```python
from build123d import *

# Parameters (mm, degrees)
BASE_FLANGE1_DEPTH        = 130
UNFOLD1_DEPTH             = 130
UNFOLD1_2_DEPTH           = 130
SKETCH6_W                 = 0.3
SKETCH6_H                 = 8
CUT_EXTRUDE1_DEPTH        = 235.985371885
LPATTERN1_COUNT           = 3
LPATTERN1_PITCH           = 11
LPATTERN2_COUNT           = 3
LPATTERN2_PITCH           = 100
LPATTERN2_COPY_1_SKETCH_W = 0.3
LPATTERN2_COPY_1_SKETCH_H = 8
LPATTERN2_COPY_1_DEPTH    = 235.985371885
LPATTERN2_COPY_2_SKETCH_W = 0.3
LPATTERN2_COPY_2_SKETCH_H = 8
LPATTERN2_COPY_2_DEPTH    = 235.985371885
LPATTERN2_COPY_3_SKETCH_W = 0.3
LPATTERN2_COPY_3_SKETCH_H = 8
LPATTERN2_COPY_3_DEPTH    = 235.985371885
LPATTERN2_COPY_4_SKETCH_W = 0.3
LPATTERN2_COPY_4_SKETCH_H = 8
LPATTERN2_COPY_4_DEPTH    = 235.985371885
FOLD1_DEPTH               = 130
FOLD1_2_DEPTH             = 130
FOLD1_START               = 30
FOLD1_3_DEPTH             = 70
FOLD1_START_2             = 8
FOLD1_4_DEPTH             = 3
FOLD1_START_3             = 19
FOLD1_5_DEPTH             = 3
FOLD1_START_4             = 108
FOLD1_6_DEPTH             = 3
FOLD1_START_5             = 119
FOLD1_7_DEPTH             = 3


# Read off the part's stored shape, not the designer's step: Unfold1, Fold1
# Sheet-metal steps are written as plain solids
with BuildPart() as part:
    # Sketch1 → Base-Flange1 (new body)
    with BuildSketch(Plane(origin=(0, 0, 0), x_dir=(1, 0, 0), z_dir=(0, 1, 0))):
        with BuildLine():
            ThreePointArc((195.5, 0), (194.920264754, 15.044613261), (193.184497308, 30))
            Line((193.184497308, 30), (193.431536307, 30.038363171))
            ThreePointArc((193.431536307, 30.038363171), (195.169523405, 15.063851897), (195.75, 0))
            Line((195.75, 0), (195.5, 0))
        make_face()
    extrude(amount=BASE_FLANGE1_DEPTH)

    # Unfold1 outline → Unfold1 (cut)
    with BuildSketch(Plane(origin=(0, 0, 0), x_dir=(1, 0, 0), z_dir=(0, 1, 0))):
        with BuildLine():
            Line((195.5, 0), (195.5, 9.890020227))
            ThreePointArc((195.5, 9.890020227), (194.726536236, 19.990962601), (193.431536307, 30.038363171))
            Line((193.431536307, 30.038363171), (193.184497308, 30))
            ThreePointArc((193.184497308, 30), (194.920264754, 15.044613261), (195.5, 0))
        make_face()
    extrude(amount=UNFOLD1_DEPTH, mode=Mode.SUBTRACT)

    # Unfold1 2 outline → Unfold1 2 (add)
    with BuildSketch(Plane(origin=(0, 0, 0), x_dir=(1, 0, 0), z_dir=(0, 1, 0))):
        with BuildLine():
            Line((195.75, 0), (195.75, 30.138261696))
            Line((195.75, 30.138261696), (195.5, 30.138261696))
            Line((195.5, 30.138261696), (195.5, 9.890020227))
            ThreePointArc((195.5, 9.890020227), (195.687490019, 4.946589737), (195.75, 0))
        make_face()
    extrude(amount=UNFOLD1_2_DEPTH)

    # Sketch6 → Cut-Extrude1 (cut, symmetric)
    with BuildSketch(Plane(origin=(195.75, 0, -195.75), x_dir=(0, 0, 1), z_dir=(-1, 0, 0))):
        with Locations((175.6, 126)):
            Rectangle(SKETCH6_W, SKETCH6_H)
    cut_extrude1 = extrude(amount=CUT_EXTRUDE1_DEPTH, both=True, mode=Mode.SUBTRACT)

    # LPattern1: Cut-Extrude1 ×3
    with Locations(*[(0, -i * LPATTERN1_PITCH, 0) for i in range(1, LPATTERN1_COUNT)]):
        add(cut_extrude1, mode=Mode.SUBTRACT)

    # LPattern2: Cut-Extrude1 ×3
    with Locations(*[(0, -i * LPATTERN2_PITCH, 0) for i in range(1, LPATTERN2_COUNT)]):
        add(cut_extrude1, mode=Mode.SUBTRACT)

    # LPattern2 copy 1 sketch → LPattern2 copy 1 (cut, symmetric)
    with BuildSketch(Plane(origin=(195.75, -111, -195.75), x_dir=(0, 0, 1), z_dir=(-1, 0, 0))):
        with Locations((175.6, 126)):
            Rectangle(LPATTERN2_COPY_1_SKETCH_W, LPATTERN2_COPY_1_SKETCH_H)
    extrude(amount=LPATTERN2_COPY_1_DEPTH, both=True, mode=Mode.SUBTRACT)

    # LPattern2 copy 2 sketch → LPattern2 copy 2 (cut, symmetric)
    with BuildSketch(Plane(origin=(195.75, -211, -195.75), x_dir=(0, 0, 1), z_dir=(-1, 0, 0))):
        with Locations((175.6, 126)):
            Rectangle(LPATTERN2_COPY_2_SKETCH_W, LPATTERN2_COPY_2_SKETCH_H)
    extrude(amount=LPATTERN2_COPY_2_DEPTH, both=True, mode=Mode.SUBTRACT)

    # LPattern2 copy 3 sketch → LPattern2 copy 3 (cut, symmetric)
    with BuildSketch(Plane(origin=(195.75, -122, -195.75), x_dir=(0, 0, 1), z_dir=(-1, 0, 0))):
        with Locations((175.6, 126)):
            Rectangle(LPATTERN2_COPY_3_SKETCH_W, LPATTERN2_COPY_3_SKETCH_H)
    extrude(amount=LPATTERN2_COPY_3_DEPTH, both=True, mode=Mode.SUBTRACT)

    # LPattern2 copy 4 sketch → LPattern2 copy 4 (cut, symmetric)
    with BuildSketch(Plane(origin=(195.75, -222, -195.75), x_dir=(0, 0, 1), z_dir=(-1, 0, 0))):
        with Locations((175.6, 126)):
            Rectangle(LPATTERN2_COPY_4_SKETCH_W, LPATTERN2_COPY_4_SKETCH_H)
    extrude(amount=LPATTERN2_COPY_4_DEPTH, both=True, mode=Mode.SUBTRACT)

    # Fold1 outline → Fold1 (cut)
    with BuildSketch(Plane(origin=(0, 0, 0), x_dir=(1, 0, 0), z_dir=(0, 1, 0))):
        with BuildLine():
            ThreePointArc((195.5, 9.890020227), (195.687490019, 4.946589737), (195.75, 0))
            Line((195.75, 0), (195.75, 30.138261696))
            Line((195.75, 30.138261696), (195.5, 30.138261696))
            Line((195.5, 30.138261696), (195.5, 9.890020227))
        make_face()
    extrude(amount=FOLD1_DEPTH, mode=Mode.SUBTRACT)

    # Fold1 2 outline → Fold1 2 (add)
    with BuildSketch(Plane(origin=(0, 0, 0), x_dir=(1, 0, 0), z_dir=(0, 1, 0))):
        with BuildLine():
            Line((194.448352042, 20.2506392), (194.697007224, 20.276535158))
            ThreePointArc((194.697007224, 20.276535158), (194.12564204, 25.165404877), (193.431536307, 30.038363171))
            Line((193.431536307, 30.038363171), (193.184497308, 30))
            ThreePointArc((193.184497308, 30), (193.877716571, 25.133265152), (194.448352042, 20.2506392))
        make_face()
        with BuildLine():
            ThreePointArc((195.5, 9.890020227), (195.179122281, 14.938966685), (194.727873277, 19.977934553))
            Line((194.727873277, 19.977934553), (194.479178675, 19.952419949))
            ThreePointArc((194.479178675, 19.952419949), (195.244627879, 9.989258456), (195.5, 0))
            Line((195.5, 0), (195.5, 9.890020227))
        make_face()
    extrude(amount=FOLD1_2_DEPTH)

    # Fold1 3 outline → Fold1 3 (add)
    with BuildSketch(Plane(origin=(0, 0, 0), x_dir=(1, 0, 0), z_dir=(0, 1, 0)).offset(FOLD1_START)):
        with BuildLine():
            ThreePointArc((194.727873277, 19.977934553), (194.712497491, 20.127240772), (194.697007224, 20.276535158))
            Line((194.697007224, 20.276535158), (194.448352042, 20.2506392))
            ThreePointArc((194.448352042, 20.2506392), (194.463822525, 20.101535484), (194.479178675, 19.952419949))
            Line((194.479178675, 19.952419949), (194.727873277, 19.977934553))
        make_face()
    extrude(amount=FOLD1_3_DEPTH)

    # Fold1 4 outline → Fold1 4 (add)
    with BuildSketch(Plane(origin=(0, 0, 0), x_dir=(1, 0, 0), z_dir=(0, 1, 0)).offset(FOLD1_START_2)):
        with BuildLine():
            ThreePointArc((194.727873277, 19.977934553), (194.712497491, 20.127240772), (194.697007224, 20.276535158))
            Line((194.697007224, 20.276535158), (194.448352042, 20.2506392))
            ThreePointArc((194.448352042, 20.2506392), (194.463822525, 20.101535484), (194.479178675, 19.952419949))
            Line((194.479178675, 19.952419949), (194.727873277, 19.977934553))
        make_face()
    extrude(amount=FOLD1_4_DEPTH)

    # Fold1 5 outline → Fold1 5 (add)
    with BuildSketch(Plane(origin=(0, 0, 0), x_dir=(1, 0, 0), z_dir=(0, 1, 0)).offset(FOLD1_START_3)):
        with BuildLine():
            ThreePointArc((194.727873277, 19.977934553), (194.712497491, 20.127240772), (194.697007224, 20.276535158))
            Line((194.697007224, 20.276535158), (194.448352042, 20.2506392))
            ThreePointArc((194.448352042, 20.2506392), (194.463822525, 20.101535484), (194.479178675, 19.952419949))
            Line((194.479178675, 19.952419949), (194.727873277, 19.977934553))
        make_face()
    extrude(amount=FOLD1_5_DEPTH)

    # Fold1 6 outline → Fold1 6 (add)
    with BuildSketch(Plane(origin=(0, 0, 0), x_dir=(1, 0, 0), z_dir=(0, 1, 0)).offset(FOLD1_START_4)):
        with BuildLine():
            ThreePointArc((194.727873277, 19.977934553), (194.712497491, 20.127240772), (194.697007224, 20.276535158))
            Line((194.697007224, 20.276535158), (194.448352042, 20.2506392))
            ThreePointArc((194.448352042, 20.2506392), (194.463822525, 20.101535484), (194.479178675, 19.952419949))
            Line((194.479178675, 19.952419949), (194.727873277, 19.977934553))
        make_face()
    extrude(amount=FOLD1_6_DEPTH)

    # Fold1 7 outline → Fold1 7 (add)
    with BuildSketch(Plane(origin=(0, 0, 0), x_dir=(1, 0, 0), z_dir=(0, 1, 0)).offset(FOLD1_START_5)):
        with BuildLine():
            ThreePointArc((194.727873277, 19.977934553), (194.712497491, 20.127240772), (194.697007224, 20.276535158))
            Line((194.697007224, 20.276535158), (194.448352042, 20.2506392))
            ThreePointArc((194.448352042, 20.2506392), (194.463822525, 20.101535484), (194.479178675, 19.952419949))
            Line((194.479178675, 19.952419949), (194.727873277, 19.977934553))
        make_face()
    extrude(amount=FOLD1_7_DEPTH)


solid = part.part
```
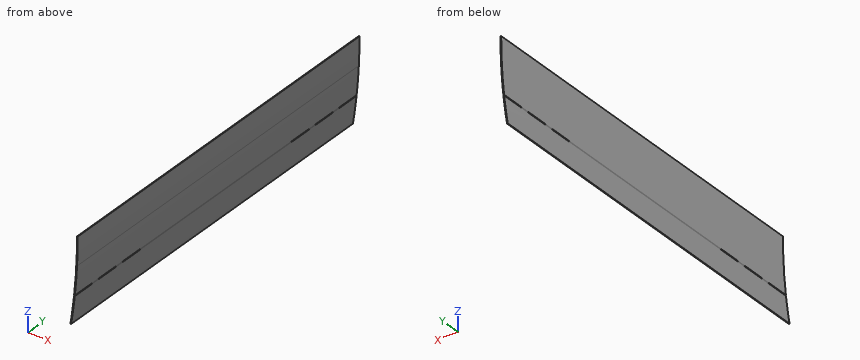
Could you check a few things on this model? Use its own coordinates, in mm. Coordinates: 2 decimals unless noted, no trailing zeros. Loops run counter-clockwise (first coordinate to the right, second up) from the corner with the lowest first, then second, coordinate; pieces in that order, holes last.
1) Imagine slicing it at A-A (y = 26.5). List the corners of the cut face in (x, z) for me.
Reported:
outline: (193.18, -30) - (193.43, -30.04) arc R195.75 ccw to (194.7, -20.28) - (194.45, -20.25) arc R195.5 cw to start; (194.48, -19.95) - (194.73, -19.98) arc R195.75 ccw to (195.75, 0) - (195.5, 0) arc R195.5 cw to start
2) Imagine slicing it at C-C (z = -15). List the corners of the cut face in (x, y) for me.
Reported:
outline: (194.92, 0) - (195.17, 0) - (195.17, 130) - (194.92, 130) - close
3) Please list where these lines run through material, in increasing order: line 1 along X through (y, z) = (38.5, -23.5); line 2 along X through (y, z) = (18, -9).
Reported:
line 1: x = 194.08 to 194.33
line 2: x = 195.29 to 195.54
4) Imagine slicing it at B-B (y = 67). List the corners of the cut face in (x, z) for me, and give its area (3 significant figures).
Reported:
outline: (193.18, -30) - (193.43, -30.04) arc R195.75 ccw to (194.7, -20.28) arc R195.75 ccw to (194.73, -19.98) arc R195.75 ccw to (195.75, 0) - (195.5, 0) arc R195.5 cw to (194.48, -19.95) arc R195.5 cw to (194.45, -20.25) arc R195.5 cw to start
area: 7.53 mm2
5) Will these pins go through, and if not, where does the flat tip stop? pin 1 Ø10 at (y, z) = (30.5, -15.5) entering from +X; pin 2 Ø6 at (y, z) = (102, -23.5) entering from -X; pin 3 Ø3 at (y, z) = (95.5, -23) entering from -X.
Reported:
pin 1: stops at x = 195.47
pin 2: stops at x = 193.7
pin 3: stops at x = 193.96
